The model under review builds one solid part; all positions refer to its coordinate system, in mm. A direction names the side the tool comes from. Round coordinates to 2 decimals unless told otherwise and drop trailing zeros. Loops run counter-clockwise (first coordinate to the right, second up) from the corner with the lowest first, then second, coordinate; pieces in that order, holes last. Notation, with made-up numbers: M 17.5,-31 L 24.5,-31 A16 ccw 24.5,-26 Z; hole C 88.25,13.5 d3. An arc over 180 degrees is marked long. Use a Markdown table: item, result. Add a question column.
```python
from build123d import *

# Parameters (mm, degrees)
SKETCH1_W                 = 32.5
SKETCH1_H                 = 42
BOSS_EXTRUDE2_DEPTH       = 3
F_2_56_TAPPED_HOLE1_D     = 1.778
F_2_56_TAPPED_HOLE1_DEPTH = 5.19583491
F_2_56_TAPPED_HOLE1_TIP   = 0.53416509
F_2_56_TAPPED_HOLE2_D     = 1.778
F_2_56_TAPPED_HOLE2_DEPTH = 5.19583491
F_2_56_TAPPED_HOLE2_TIP   = 0.53416509
CUT_EXTRUDE1_DEPTH        = 3
F_1_4_20_TAPPED_HOLE1_D   = 5.1054


with BuildPart() as part:
    # Sketch1 → Boss-Extrude2 (new body)
    with BuildSketch(Plane.XY):
        with Locations((16.25, 21)):
            Rectangle(SKETCH1_W, SKETCH1_H)
    extrude(amount=BOSS_EXTRUDE2_DEPTH)

    # #2-56 Tapped Hole1
    with Locations(Plane.ZY):
        with Locations((1.5, 33), (1.5, 9)):
            Hole(F_2_56_TAPPED_HOLE1_D / 2, depth=F_2_56_TAPPED_HOLE1_DEPTH)
            with Locations((0, 0, -(F_2_56_TAPPED_HOLE1_DEPTH + F_2_56_TAPPED_HOLE1_TIP / 2))):  # 118° drill point
                Cone(0, F_2_56_TAPPED_HOLE1_D / 2, F_2_56_TAPPED_HOLE1_TIP, mode=Mode.SUBTRACT)

    # #2-56 Tapped Hole2
    with Locations(Plane(origin=(32.5, 0, 0), x_dir=(0, 0, -1), z_dir=(1, 0, 0))):
        with Locations((-1.5, 33), (-1.5, 9)):
            Hole(F_2_56_TAPPED_HOLE2_D / 2, depth=F_2_56_TAPPED_HOLE2_DEPTH)
            with Locations((0, 0, -(F_2_56_TAPPED_HOLE2_DEPTH + F_2_56_TAPPED_HOLE2_TIP / 2))):  # 118° drill point
                Cone(0, F_2_56_TAPPED_HOLE2_D / 2, F_2_56_TAPPED_HOLE2_TIP, mode=Mode.SUBTRACT)

    # Sketch9 → Cut-Extrude1 (cut)
    with BuildSketch(Plane(origin=(0, 0, 0), x_dir=(-1, 0, 0), z_dir=(0, 0, -1))):
        with BuildLine():
            ThreePointArc((-11.4, 21), (-8.4, 18), (-5.4, 21))
            Line((-5.4, 21), (-8.4, 21))
            Line((-8.4, 21), (-11.4, 21))
        make_face()
        with BuildLine():
            Line((-8.4, 21), (-5.4, 21))
            ThreePointArc((-5.4, 21), (-8.4, 24), (-11.4, 21))
            Line((-11.4, 21), (-8.4, 21))
        make_face()
    extrude(amount=-CUT_EXTRUDE1_DEPTH, mode=Mode.SUBTRACT)

    # 1/4-20 Tapped Hole1 (through all)
    with Locations(Plane(origin=(0, 0, 0), x_dir=(-1, 0, 0), z_dir=(0, 0, -1))):
        with Locations((-16.25, 21)):
            Hole(F_1_4_20_TAPPED_HOLE1_D / 2)


solid = part.part
```
(1) For faces 1 (the face through (29.87, 9.88, 1.38)), 2 (the face through (0, 21, 1)), 3 (the face through (2.63, 9.88, 1.62)), list the 3-axis set-ups (+Z, -Z, +X, -X, +Y, -Y) from which the entire face can be reached by the end or side of a thin tool; tool diameter is ignored.
(2) Draft analysis for pull direction Y (two halves, no side actions). For faces 4 (the face through (2.63, 32.21, 1.09)), 5 (the face through (20, 21, 0)), 6 (the face through (16, 0, 1)), state which applies: released by +Y, released by -Y, zero draft, split by the parting line, or undercut.
(3) Consider section A-A, the plane x = 16.25. Give the boundary of the cut face in (y, z).
(4) Consider section C-C, the plane x = 2. Give the boundary of the cut face in (y, z), then the cut area to 3 significant figures.
(5) Consider section B-B, the plane y = 21. Give the boundary of the cut face in (x, z).
(6) To check wall thickness, follow probe 1 along Y at (x, z) = (1.7, 1.5); probe 2 along Y at (x, z) = (31, 0.9); probe 3 along X at (y, z) = (22.5, 1.15). State the ranges of each line that lie inside material, in increasing order.
(7) Consider section D-D, the plane x = 8.4. Give the boundary of the cut face in (y, z), then the cut area to 3 significant figures.
(8) Insertion check: pin 1 Ø1.6 at (y, z) = (9, 1.5) entering from -X; pin 2 Ø1.6 at (y, z) = (33, 1.5) entering from +X. Each pin has a flat end and moves straight along its axis. Give the tip position at first contact, or say it passes through.
Found:
| question | item | result |
|---|---|---|
| 1 | face 1 | +X |
| 1 | face 2 | +Z, -Z, -X, +Y, -Y |
| 1 | face 3 | -X |
| 2 | face 4 | undercut |
| 2 | face 5 | zero draft |
| 2 | face 6 | released by -Y |
| 3 | outline | M 0,0 L 18.45,0 L 18.45,3 L 0,3 Z; M 23.55,0 L 42,0 L 42,3 L 23.55,3 Z |
| 4 | outline | M 0,0 L 42,0 L 42,3 L 0,3 Z; hole C 9,1.5 d1.78; hole C 33,1.5 d1.78 |
| 4 | area | 121 mm^2 |
| 5 | outline | M 0,0 L 5.4,0 L 5.4,3 L 0,3 Z; M 11.4,0 L 13.7,0 L 13.7,3 L 11.4,3 Z; M 18.8,0 L 32.5,0 L 32.5,3 L 18.8,3 Z |
| 6 | probe 1 | y = 0 to 8.11, 9.89 to 32.11, 33.89 to 42 |
| 6 | probe 2 | y = 0 to 8.34, 9.66 to 32.34, 33.66 to 42 |
| 6 | probe 3 | x = 0 to 5.8, 11 to 14.18, 18.32 to 32.5 |
| 7 | outline | M 0,0 L 18,0 L 18,3 L 0,3 Z; M 24,0 L 42,0 L 42,3 L 24,3 Z |
| 7 | area | 108 mm^2 |
| 8 | pin 1 | stops at x = 5.25 |
| 8 | pin 2 | stops at x = 27.25 |
